Check sheet for the modelled part. Datum: model origin and axes. Units: mm. Coordinates: 2 decimals unless noted, no trailing zeros. Loops run counter-clockwise (first coordinate to the right, second up) from the corner with the lowest first, then second, coordinate; pieces in that order, holes last. Notation, with made-up numbers: (85, -0.75) -> (111, -0.75) arc R5 cw to (111, 4.25) -> close; hole circle Ø11 at (20.25, 18.25). An arc over 180 degrees is marked (long way). Use one line per item in the form item = value.
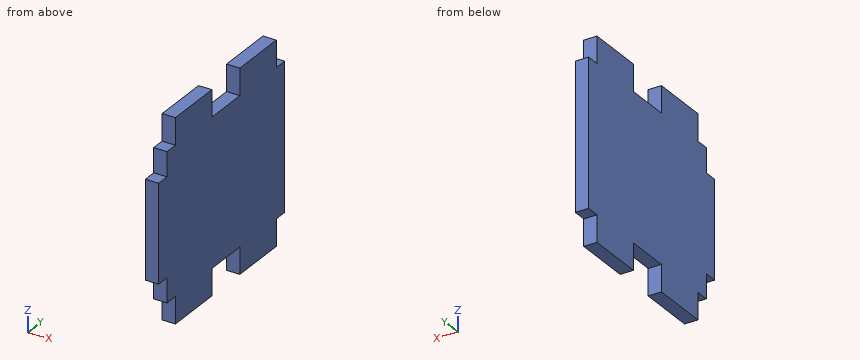
Autodesk Inventor part; units mm, degrees
ref_plane "YZ Plane" through (0, 0, 0) normal (1, 0, 0) x (0, 1, 0)
ref_plane "XZ Plane" through (0, 0, 0) normal (0, 1, 0) x (-1, 0, 0)
ref_plane "XY Plane" through (0, 0, 0) normal (0, 0, 1) x (1, 0, 0)
sketch "Sketch2" plane through (0, 0, 0) normal (1, 0, 0) x (0, 1, 0)
  line L0 (21, -16.5) -> (18, -16.5)
  line L1 (-21, -16.5) -> (-21, -11)
  line L2 (-21, 16.5) -> (-18, 16.5)
  line L3 (21, 16.5) -> (21, -16.5)
  line L4 (21, -16.5) -> (-21, 16.5) construction
  line L5 (-21, -16.5) -> (21, 16.5) construction
  line L6 (0, -31.5) -> (0, 31.5) construction
  line L7 (-33, 0) -> (30, 0) construction
  line L8 (18, 16.5) -> (18, 22.5)
  line L9 (18, 22.5) -> (5, 22.5)
  line L10 (5, 22.5) -> (5, 16.5)
  line L11 (18, 16.5) -> (21, 16.5)
  line L12 (5, 16.5) -> (18, 16.5)
  line L13 (0, 16.5) -> (5, 16.5)
  line L14 (-18, 16.5) -> (-18, 22.5)
  line L15 (-18, 22.5) -> (-5, 22.5)
  line L16 (-5, 22.5) -> (-5, 16.5)
  line L17 (18, -16.5) -> (5, -16.5)
  line L18 (5, -16.5) -> (-5, -16.5)
  line L19 (-5, -16.5) -> (-18, -16.5)
  line L20 (-18, -16.5) -> (-21, -16.5)
  line L21 (-18, 16.5) -> (-5, 16.5)
  line L22 (-5, 16.5) -> (0, 16.5)
  line L23 (-21, 11) -> (-24, 11)
  line L24 (-24, 11) -> (-24, -11)
  line L25 (-24, -11) -> (-21, -11)
  line L26 (-21, 11) -> (-21, 16.5)
  line L27 (-21, -11) -> (-21, 11)
  line L28 (18, -16.5) -> (18, -22.5)
  line L29 (18, -22.5) -> (5, -22.5)
  line L30 (5, -22.5) -> (5, -16.5)
  line L31 (-5, -16.5) -> (-5, -22.5)
  line L32 (-5, -22.5) -> (-18, -22.5)
  line L33 (-18, -22.5) -> (-18, -16.5)
  point P0 (0, 0)
  dimension "d4" = 42
  dimension "d5" = 33
  dimension "d9" = 6
  dimension "d11" = 3
  dimension "d12" = 22
  dimension "d13" = 6
  dimension "d16" = 3
  dimension "d17" = 5
extrude "Extrusion2" add sketch "Sketch2" against normal blind 3
equation "\"d12\" = 0.666667 * d5"
properties part number "X-Motor-Housing_Motor-Side"
(1) Scan lines: line 1 along Y through (x, z) = (-1.4, 18); line 2 along Z through (x, y) = (-0.5, 2.5). Record each from-to range of solid material in increasing order.
Established:
line_1 = -18 to -5, 5 to 18
line_2 = -16.5 to 16.5
(2) Section check B-B, the plane x = -2.05. Record the boundary of the cut face in (y, z).
Established:
outline = (-24, -11) -> (-21, -11) -> (-21, -16.5) -> (-18, -16.5) -> (-18, -22.5) -> (-5, -22.5) -> (-5, -16.5) -> (5, -16.5) -> (5, -22.5) -> (18, -22.5) -> (18, -16.5) -> (21, -16.5) -> (21, 16.5) -> (18, 16.5) -> (18, 22.5) -> (5, 22.5) -> (5, 16.5) -> (-5, 16.5) -> (-5, 22.5) -> (-18, 22.5) -> (-18, 16.5) -> (-21, 16.5) -> (-21, 11) -> (-24, 11) -> close
(3) Section check D-D, the plane z = 13. Record the boundary of the cut face in (x, y), plus the area to 3 significant figures.
Established:
outline = (-3, -21) -> (0, -21) -> (0, 21) -> (-3, 21) -> close
area = 126 mm²
(4) Section check A-A, the plane z = -18.5. Record the boundary of the cut face in (x, y).
Established:
outline = (-3, -18) -> (0, -18) -> (0, -5) -> (-3, -5) -> close; (-3, 5) -> (0, 5) -> (0, 18) -> (-3, 18) -> close
(5) Section check C-C, the plane y = -2.5. Record the boundary of the cut face in (x, z), plus the area to 3 significant figures.
Established:
outline = (-3, -16.5) -> (0, -16.5) -> (0, 16.5) -> (-3, 16.5) -> close
area = 99.0 mm²
(6) Go/stop test with flat-tipped pins: P1, Ø1.5, axis at x = -2, z = -14.5, coming from the -Y side; P2, Ø1.5, axis at x = -2, y = 2, coming from the +Z side; P3, Ø1.5, axis at x = -1.5, z = -20.5, coming from the -Y side. Record where each tip stops, or that it passes through.
Established:
P1 = -21
P2 = 16.5
P3 = -18
